from build123d import *

# Parameters (mm, degrees)
SKETCH1_R           = 0.5
BOSS_EXTRUDE1_DEPTH = 2


with BuildPart() as part:
    # Sketch1 → Boss-Extrude1 (new body)
    with BuildSketch(Plane.XY):
        with BuildLine():
            Line((-3.617777686, 53.531365908), (-8.799601245, 42.545043716))
            ThreePointArc((-8.799601245, 42.545043716), (-9.122569183, 40.152730346), (-8.010250683, 38.010250683))
            Line((-8.010250683, 38.010250683), (-6.171572875, 36.171572875))
            ThreePointArc((-6.171572875, 36.171572875), (-5.30448187, 34.87387948), (-5, 33.343145751))
            Line((-5, 33.343145751), (-5, -33.343145751))
            ThreePointArc((-5, -33.343145751), (-5.30448187, -34.87387948), (-6.171572875, -36.171572875))
            Line((-6.171572875, -36.171572875), (-8.010250683, -38.010250683))
            ThreePointArc((-8.010250683, -38.010250683), (-9.122569183, -40.152730346), (-8.799601245, -42.545043716))
            Line((-8.799601245, -42.545043716), (-3.617777686, -53.531365908))
            ThreePointArc((-3.617777686, -53.531365908), (0, -55.825), (3.617777686, -53.531365908))
            Line((3.617777686, -53.531365908), (8.799601245, -42.545043716))
            ThreePointArc((8.799601245, -42.545043716), (9.122569183, -40.152730346), (8.010250683, -38.010250683))
            Line((8.010250683, -38.010250683), (6.171572875, -36.171572875))
            ThreePointArc((6.171572875, -36.171572875), (5.30448187, -34.87387948), (5, -33.343145751))
            Line((5, -33.343145751), (5, 33.343145751))
            ThreePointArc((5, 33.343145751), (5.30448187, 34.87387948), (6.171572875, 36.171572875))
            Line((6.171572875, 36.171572875), (8.010250683, 38.010250683))
            ThreePointArc((8.010250683, 38.010250683), (9.122569183, 40.152730346), (8.799601245, 42.545043716))
            Line((8.799601245, 42.545043716), (3.617777686, 53.531365908))
            ThreePointArc((3.617777686, 53.531365908), (0, 55.825), (-3.617777686, 53.531365908))
        make_face()
        with Locations((-5, 40)):
            Circle(SKETCH1_R, mode=Mode.SUBTRACT)
        with Locations(Location((5, 40, 0), (0, 0, 180))):
            Circle(SKETCH1_R, mode=Mode.SUBTRACT)
        with Locations((5, -40)):
            Circle(SKETCH1_R, mode=Mode.SUBTRACT)
        with Locations(Location((-5, -40, 0), (0, 0, 180))):
            Circle(SKETCH1_R, mode=Mode.SUBTRACT)
    extrude(amount=BOSS_EXTRUDE1_DEPTH)


solid = part.part
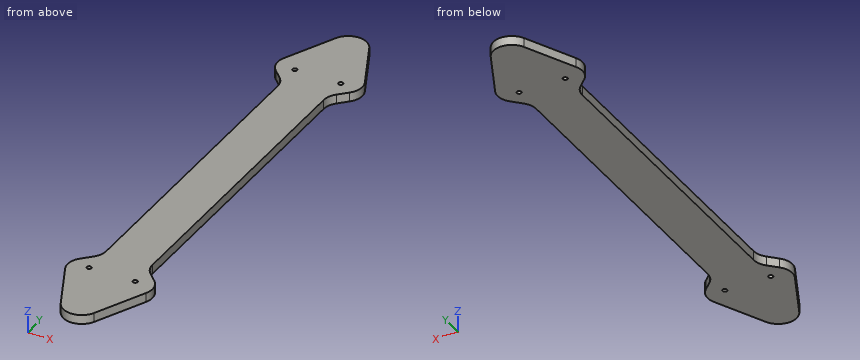
Geometry: final body of the model. Coordinates: model frame, mm. Round coordinates to 2 decimals unless told otherwise and drop trailing zeros. Order: outer loops, then holes, each group sorted by start corner. A loop starts at its lowest first (then second) coordinate and runs counter-clockwise, first axis right, second up. Notation, with made-up numbers: (56.5, -20.5) -> (87.5, -20.5) arc R31 ccw to (87.5, 15.5) -> close; hole circle Ø5 at (-20, 79). An arc over 180 degrees is marked (long way). Put each result on its own line as item: value. Start each with the question number.
Q1. Section B-B on y = -49. Return the cut outline in (x, z).
Q2. Line query: probe 1 along X at (y, z) = (-40, 0.85); probe 2 along Y at (x, z) = (7, 1.15); probe 3 along X at (y, z) = (-18.5, 1.6). Output: solid intervals per line, ascending.
Q3. First-contact query: pin 1 (1 mm diameter, centred on y = 20.5, z = 0.5, fed in from +X). Flat tip, straight axial feed; report the tip coordinate or a pass-through.
Q4. Section A-A on y = 5.5. Return the cut outline in (x, z).
Ans:
1. outline: (-5.76, 0) -> (5.76, 0) -> (5.76, 2) -> (-5.76, 2) -> close
2. probe 1: x = -9.09 to -5.5, -4.5 to 4.5, 5.5 to 9.09
2. probe 2: y = -46.36 to -37, 37 to 46.36
2. probe 3: x = -5 to 5
3. pin 1: stops at x = 5
4. outline: (-5, 0) -> (5, 0) -> (5, 2) -> (-5, 2) -> close
